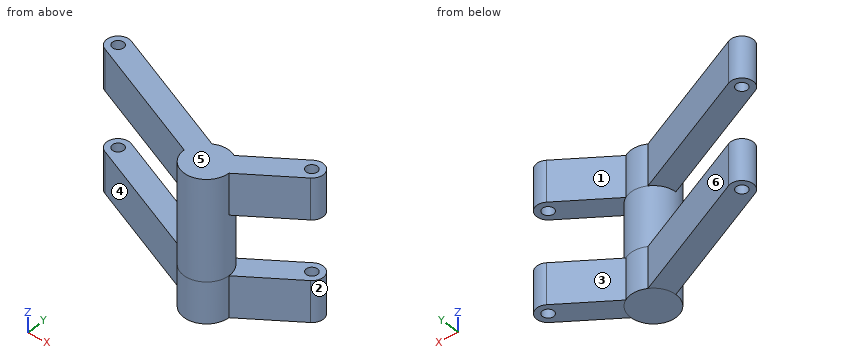
from build123d import *
from build123d.topology import SkipClean

# Parameters (mm, degrees)
SKETCH1_R           = 5
BOSS_EXTRUDE3_DEPTH = 6.5
BOSS_EXTRUDE4_START = 9
SKETCH3_R           = 1.25
SKETCH3_R_2         = 5
BOSS_EXTRUDE4_DEPTH = 9


with BuildPart() as part:
    # Sketch1 → Boss-Extrude3 (new, symmetric)
    with BuildSketch(Plane.XY):
        with Locations(Location((0, 0, 0), (0, 0, 180))):
            Circle(SKETCH1_R)
    extrude(amount=BOSS_EXTRUDE3_DEPTH, both=True)

    # Sketch3 → Boss-Extrude4 (add)
    # profile 1 of 3: a face of its own
    with BuildSketch(Plane.XY.offset(6.5).offset(BOSS_EXTRUDE4_START)):
        with BuildLine():
            ThreePointArc((2.483058563, 4.339864073), (4.325233682, 2.508456416), (5, 0))
            Line((5, 0), (16.427426363, 7.947573637))
            ThreePointArc((16.427426363, 7.947573637), (17.052426363, 11.427426363), (13.572573637, 12.052426363))
            Line((13.572573637, 12.052426363), (2.483058563, 4.339864073))
        make_face()
        with Locations((15, 10)):
            Circle(SKETCH3_R, mode=Mode.SUBTRACT)
    # profile 2 of 3: a face of its own
    with BuildSketch(Plane.XY.offset(6.5).offset(BOSS_EXTRUDE4_START)):
        with BuildLine():
            Line((-33.518152484, 12.716720446), (-5, 0))
            ThreePointArc((-5, 0), (-4.321713979, 2.514515517), (-2.470884686, 4.346806744))
            Line((-2.470884686, 4.346806744), (-31.481847516, 17.283279554))
            ThreePointArc((-31.481847516, 17.283279554), (-34.783279554, 16.018152484), (-33.518152484, 12.716720446))
        make_face()
        with Locations((-32.5, 15)):
            Circle(SKETCH3_R, mode=Mode.SUBTRACT)
    # profile 3 of 3: a face of its own
    with BuildSketch(Plane.XY.offset(6.5).offset(BOSS_EXTRUDE4_START)):
        Circle(SKETCH3_R_2)
    boss_extrude4 = extrude(amount=-BOSS_EXTRUDE4_DEPTH)

    # Mirror12: Boss-Extrude4 across plane
    with SkipClean():  # the faces are left unmerged after this step: merging them gives an invalid solid
        add(boss_extrude4.mirror(Plane.XY))


solid = part.part
The listing builds one solid part. Answer for the finished solid, in the listing's coordinates (mm). Face numbers are marked on the shaded views. A direction names the side the tool comes from. Round coordinates to 2 decimals unless told otherwise and drop trailing zeros. Write each loop counter-clockwise with the first axis right and the second up, starting at its lowest first coordinate (ties: lowest second). Pieces come first, ordered by that corner, then holes. Notation, with made-up numbers: M 60,84 L 106,84 A36 ccw 106,121 Z; hole C 26.5,41 d7. An arc over 180 degrees is marked long. Write each question's results on one line, items separated by ' | '. Start each with the question number.
Item 1: A cutting plane is placed at A-A on x = 15. Write down the section's boundary in (y, z).
Item 2: For the marked faces 1 and 2, determine the directions among +Z, -Z, +X, -X, +Y, -Y from which every point of the face is accessible in a straight line to the end or side of a thin tool.
Item 3: A cutting plane is placed at B-B on y = 15. Write down the section's boundary in (x, z).
Item 4: A cutting plane is placed at C-C on z = 8.5. Write down the section's boundary in (x, y).
Item 5: For a pull along X with two mould halves and no side action, classify the marked faces 3, 4, 5 and 6 as pulls with the +X half, pulls with the -X half, needs draft (parallel to the pull), parting line crosses it, or undercut.
Item 6: Straight lines are drawn through the part: L1, parallel to Z at x = -16.5, y = 9; L2, parallel to Y at x = 15, z = -12.75; L3, parallel to X at y = 12, z = -11. For each, find the intervals that lie inside material, in ascending order. Write a range as [from, to].
Item 7: Flat-ended cylindrical pins translate along their axes: pin 1 Ø2 at (x, y) = (15, 10) entering from -Z; pin 2 Ø8 at (y, z) = (4, 9) entering from +X; pin 3 Ø2 at (x, z) = (-6, -7.5) entering from +Y; pin 4 Ø2 at (y, z) = (1.5, -12.5) entering from +X. Find the tip coordinate at first contact, or state that the pin passes through.
Item 8: A cutting plane is placed at D-D on y = 10. Write down the section's boundary in (x, z), and give its area (3 significant figures).
Check sheet entries:
1) outline: M 6.95,-15.5 L 8.75,-15.5 L 8.75,-6.5 L 6.95,-6.5 Z; M 6.95,6.5 L 8.75,6.5 L 8.75,15.5 L 6.95,15.5 Z; M 11.25,-15.5 L 12.5,-15.5 L 12.5,-6.5 L 11.25,-6.5 Z; M 11.25,6.5 L 12.5,6.5 L 12.5,15.5 L 11.25,15.5 Z
2) face 1: +Z, -Z, +Y | face 2: +Z, -Z
3) outline: M -35,-15.5 L -33.75,-15.5 L -33.75,-6.5 L -35,-6.5 Z; M -35,6.5 L -33.75,6.5 L -33.75,15.5 L -35,15.5 Z; M -31.25,-15.5 L -26.36,-15.5 L -26.36,-6.5 L -31.25,-6.5 Z; M -31.25,6.5 L -26.36,6.5 L -26.36,15.5 L -31.25,15.5 Z
4) outline: M -33.52,12.72 L -5,0 A5 ccw 5,0 L 16.43,7.95 A2.5 ccw 13.57,12.05 L 2.48,4.34 A5 ccw -2.47,4.35 L -31.48,17.28 A2.5 ccw Z; hole C -32.5,15 d2.5; hole C 15,10 d2.5
5) face 3: undercut | face 4: pulls with the -X half | face 5: needs draft | face 6: undercut
6) L1: [-15.5, -6.5], [6.5, 15.5] | L2: [6.95, 8.75], [11.25, 12.5] | L3: [-31.91, -19.63], [13.5, 16.5]
7) pin 1: through | pin 2: x = 16.5 | pin 3: y = 6.37 | pin 4: x = 8.59
8) outline: M -27.43,-15.5 L -15.15,-15.5 L -15.15,-6.5 L -27.43,-6.5 Z; M -27.43,6.5 L -15.15,6.5 L -15.15,15.5 L -27.43,15.5 Z; M 10.62,-15.5 L 13.75,-15.5 L 13.75,-6.5 L 10.62,-6.5 Z; M 10.62,6.5 L 13.75,6.5 L 13.75,15.5 L 10.62,15.5 Z; M 16.25,-15.5 L 17.5,-15.5 L 17.5,-6.5 L 16.25,-6.5 Z; M 16.25,6.5 L 17.5,6.5 L 17.5,15.5 L 16.25,15.5 Z | area: 300 mm²
